Read the model definition and answer for the solid it produces. Units are mm, in the model's axes. Face numbers are marked on the shaded views. A direction names the side the tool comes from. Give positions to 0.01 mm unless a question says otherwise; leave off trailing zeros. Order: outer loops, then holes, each group sorted by start corner. A loop starts at its lowest first (then second) coordinate and runs counter-clockwise, first axis right, second up.
Item 1: A cutting plane is placed at A-A (x = -49). Write down the section's boundary in (y, z), plus the area to 3 significant figures.
Item 2: A cutting plane is placed at D-D (x = -16.5). Write down the section's boundary in (y, z), plus the area to 3 significant figures.
Item 3: Given pin 1 Ø17.5 at (x, z) = (-11.5, -19.92) entering from -Y; pin 2 Ø10 at (y, z) = (3.5, -34.5) entering from -X; pin 3 Ø9 at (x, z) = (34.972, -25.9) entering from -Y, each flat-ended and moving along its own axis, determine where each tip first touches the part or whether it passes through.
Item 4: Find the intervals of material crossed by line 1 along Z through (x, y) = (-34.5, 6.25); line 2 along X through (y, z) = (20, -22), in increasing order.
Item 5: Which of the six approach directions +Z, -Z, +X, -X, +Y, -Y give full straight-line access (tool end or side, diameter ignored) to the marked faces 1 and 2?
Item 6: A cutting plane is placed at C-C (y = 6.25). State how many separate pieces and enclosed holes the cut face has, plus the area to 3 significant figures.
Item 7: A cutting plane is placed at B-B (z = 6). Write down the section's boundary in (x, y).
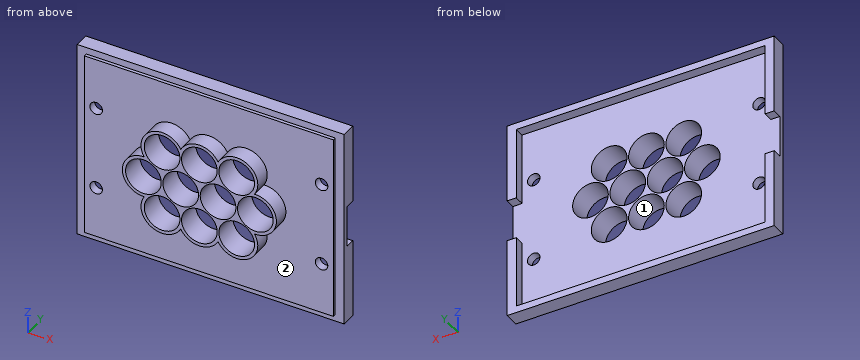
Autodesk Inventor part; units mm, degrees
ref_plane "YZ Plane" through (0, 0, 0) normal (1, 0, 0) x (0, 1, 0)
ref_plane "XZ Plane" through (0, 0, 0) normal (0, 1, 0) x (-1, 0, 0)
ref_plane "XY Plane" through (0, 0, 0) normal (0, 0, 1) x (1, 0, 0)
sketch "Sketch1" plane through (0, 0, 0) normal (0, 1, 0) x (-1, 0, 0)
  circle A0 centre (0, 0) radius 11
  line L0 (11, 0.0002) -> (12, 0.0002) construction
  circle A1 centre (23, 0) radius 11
  line L1 (34, 0) -> (35, 0) construction
  circle A2 centre (46, 0) radius 11
  line L2 (57, 0) -> (58, 0) construction
  circle A3 centre (69, 0) radius 11
  line L3 (34.5, 0) -> (34.5, -17.154) construction
  line L4 (34.5, 0) -> (34.5, 17.658) construction
  line L5 (55, 12.6387) -> (55, -13.5831) construction
  line L6 (55, 12.6387) -> (55, 17.658) construction
  line L7 (55, -13.5831) -> (55, -17.154) construction
  line L8 (11.5, 0.0002) -> (11.5, -16.2579) construction
  line L9 (11.5, 0.0002) -> (11.5, 19.9186) construction
  circle A4 centre (0, 0) radius 12 construction
  circle A5 centre (23, 0) radius 12 construction
  circle A6 centre (46, 0) radius 12 construction
  circle A7 centre (69, 0) radius 12 construction
  circle A8 centre (11.5, 19.9186) radius 11
  circle A9 centre (34.5, 19.9186) radius 11
  circle A10 centre (11.5, -19.9186) radius 11
  circle A11 centre (57.5, 19.9186) radius 11
  circle A12 centre (57.5, -19.9186) radius 12 construction
  circle A13 centre (34.5, -19.9186) radius 12 construction
  circle A14 centre (11.5, 19.9186) radius 12 construction
  circle A15 centre (34.5, 19.9186) radius 12 construction
  circle A16 centre (57.5, 19.9186) radius 12 construction
  line L10 (11.5, 19.9186) -> (57.5, 19.9186) construction
  arc A17 (2.3131, -12.7926) -> (0.5, -12.9904) centre (0, 0) ccw construction
  circle A18 centre (11.5, 19.9186) radius 13 construction
  circle A19 centre (34.5, 19.9186) radius 13 construction
  circle A20 centre (57.5, 19.9186) radius 13 construction
  circle A21 centre (69, 0) radius 13 construction
  circle A22 centre (57.5, -19.9186) radius 13 construction
  circle A23 centre (34.5, -19.9186) radius 13 construction
  arc A24 (0.5, 12.9904) -> (0.5, -12.9904) centre (0, 0) ccw
  line L11 (57.5, -19.9186) -> (11.5, -19.9186) construction
  circle A25 centre (11.5, -19.9186) radius 13 construction
  arc A26 (0.5, -12.9904) -> (23, -25.9808) centre (11.5, -19.9186) ccw
  arc A27 (23, -25.9808) -> (46, -25.9808) centre (34.5, -19.9186) ccw
  arc A28 (46, -25.9808) -> (68.5, -12.9904) centre (57.5, -19.9186) ccw
  arc A29 (68.5, -12.9904) -> (68.5, 12.9904) centre (69, 0) ccw
  arc A30 (68.5, 12.9904) -> (46, 25.9808) centre (57.5, 19.9186) ccw
  arc A31 (46, 25.9808) -> (23, 25.9808) centre (34.5, 19.9186) ccw
  arc A32 (23, 25.9808) -> (0.5, 12.9904) centre (11.5, 19.9186) ccw
  circle A33 centre (11.5, -19.9186) radius 12 construction
  circle A34 centre (34.5, -19.9186) radius 11
  circle A35 centre (57.5, -19.9186) radius 11
  dimension "d0" = 22
  dimension "d6" = 22
  dimension "d1" = 1
  dimension "d2" = 22
  dimension "d3" = 1
  dimension "d4" = 22
  dimension "d5" = 1
  dimension "d7" = 24
  dimension "d8" = 24
  dimension "d9" = 24
  dimension "d10" = 24
  dimension "d11" = 22
  dimension "d12" = 22
  dimension "d16" = 22
  dimension "d17" = 22
  dimension "d19" = 24
  dimension "d21" = 24
  dimension "d22" = 24
  dimension "d23" = 24
  dimension "d25" = 26
  dimension "d27" = 26
  dimension "d28" = 26
  dimension "d29" = 26
  dimension "d30" = 26
  dimension "d31" = 26
  dimension "d32" = 26
  dimension "d33" = 26
  dimension "d67" = 24
  dimension "d71" = 24
  dimension "d72" = 22
  dimension "d73" = 22
extrude "Extrusion1" add sketch "Sketch1" along normal blind 15
sketch "Sketch2" plane through (0, 15, 0) normal (0, 1, 0) x (1, 0, 0)
  circle A0 centre (-23, 0) radius 11
  circle A1 centre (-46, 0) radius 11
  line L0 (-35, 0) -> (-34, 0) construction
  line L1 (-111.2, 57.65) -> (42.2, 57.65)
  line L2 (42.2, 57.65) -> (42.2, -57.65)
  line L3 (42.2, -57.65) -> (-111.2, -57.65)
  line L4 (-111.2, -57.65) -> (-111.2, 57.65)
  line L5 (-111.2, 57.65) -> (42.2, -57.65) construction
  line L6 (42.2, 57.65) -> (-111.2, -57.65) construction
  arc A2 (-46, 25.9808) -> (-68.5, 12.9904) centre (-57.5, 19.9186) ccw
  arc A3 (-23, 25.9808) -> (-46, 25.9808) centre (-34.5, 19.9186) ccw
  arc A4 (-0.5, 12.9904) -> (-23, 25.9808) centre (-11.5, 19.9186) ccw
  arc A5 (-0.5, -12.9904) -> (-0.5, 12.9904) centre (0, 0) ccw
  arc A6 (-23, -25.9808) -> (-0.5, -12.9904) centre (-11.5, -19.9186) ccw
  arc A7 (-46, -25.9808) -> (-23, -25.9808) centre (-34.5, -19.9186) ccw
  arc A8 (-68.5, -12.9904) -> (-46, -25.9808) centre (-57.5, -19.9186) ccw
  arc A9 (-68.5, 12.9904) -> (-68.5, -12.9904) centre (-69, 0) ccw
  arc A10 (-69, 13) -> (-68.5, -12.9904) centre (-69, 0) ccw
  arc A11 (-46, 25.9808) -> (-68.5, 12.9904) centre (-57.5, 19.9186) ccw
  arc A12 (-23, 25.9808) -> (-46, 25.9808) centre (-34.5, 19.9186) ccw
  arc A13 (-0.5, 12.9904) -> (-23, 25.9808) centre (-11.5, 19.9186) ccw
  arc A14 (-0.5, -12.9904) -> (-0.5, 12.9904) centre (0, 0) ccw
  arc A15 (-23, -25.9808) -> (-0.5, -12.9904) centre (-11.5, -19.9186) ccw
  arc A16 (-46, -25.9808) -> (-23, -25.9808) centre (-34.5, -19.9186) ccw
  arc A17 (-68.5, -12.9904) -> (-46, -25.9808) centre (-57.5, -19.9186) ccw
  arc A18 (-68.5, 12.9904) -> (-68.5, -12.9904) centre (-69, 0) ccw
  point P0 (-34.5, 0)
  dimension "d36" = 115.3
  dimension "d37" = 153.4
extrude "Extrusion2" add sketch "Sketch2" against normal blind 5 contours L1 L2 L3 L4
sketch "Sketch3" plane through (0, 15, 0) normal (0, 1, 0) x (1, 0, 0)
  line L0 (42.2, 57.65) -> (-111.2, 57.65)
  line L1 (42.2, -57.65) -> (42.2, 57.65)
  line L2 (-111.2, -57.65) -> (42.2, -57.65)
  line L3 (-111.2, 57.65) -> (-111.2, -57.65)
  line L4 (-111.2, -57.65) -> (42.2, -57.65)
  line L5 (42.2, -57.65) -> (42.2, 57.65)
  line L6 (42.2, 57.65) -> (-111.2, 57.65)
  line L7 (-111.2, 57.65) -> (-111.2, -57.65)
  circle A0 centre (-57.5, -19.9186) radius 11
  circle A1 centre (-11.5, 19.9186) radius 11
  circle A2 centre (-34.5, -19.9186) radius 11
  circle A3 centre (-11.5, -19.9186) radius 11
  circle A4 centre (-69, 0) radius 11
  circle A5 centre (-46, 0) radius 11
  circle A6 centre (-23, 0) radius 11
  circle A7 centre (0, 0) radius 11
  line L8 (-116.8026, 61.8611) -> (47.8026, 61.8611)
  line L9 (47.8026, 61.8611) -> (47.8026, -61.8611)
  line L10 (47.8026, -61.8611) -> (-116.8026, -61.8611)
  line L11 (-116.8026, -61.8611) -> (-116.8026, 61.8611)
  line L12 (-116.8026, 61.8611) -> (47.8026, -61.8611) construction
  line L13 (47.8026, 61.8611) -> (-116.8026, -61.8611) construction
  line L14 (-111.2, -57.65) -> (42.2, -57.65)
  line L15 (42.2, -57.65) -> (42.2, 57.65)
  line L16 (42.2, 57.65) -> (-111.2, 57.65)
  line L17 (-111.2, 57.65) -> (-111.2, -57.65)
  line L18 (-111.2, -57.65) -> (42.2, 57.65) construction
  line L19 (42.2, -57.65) -> (-111.2, 57.65) construction
  point P0 (-34.5, 0)
extrude "Extrusion3" add sketch "Sketch3" along normal blind 6 and the other way blind 3 contours L8 L9 L10 L11
sketch "Sketch4" plane through (0, 15, 0) normal (0, 1, 0) x (1, 0, 0)
  line L0 (-111.2, -57.65) -> (42.2, -57.65)
  line L1 (42.2, -57.65) -> (42.2, 57.65)
  line L2 (42.2, 57.65) -> (-111.2, 57.65)
  line L3 (-111.2, 57.65) -> (-111.2, -57.65)
  circle A0 centre (-57.5, -19.9186) radius 11
  circle A1 centre (-11.5, 19.9186) radius 11
  circle A2 centre (-34.5, -19.9186) radius 11
  circle A3 centre (-11.5, -19.9186) radius 11
  circle A4 centre (-69, 0) radius 11
  circle A5 centre (-46, 0) radius 11
  circle A6 centre (-23, 0) radius 11
  circle A7 centre (0, 0) radius 11
  line L4 (-111.2, 57.65) -> (-103.972, 57.65) construction
  line L5 (-103.972, 57.65) -> (-103.972, 25.9) construction
  line L6 (-103.972, 25.9) -> (-111.2, 25.9) construction
  line L7 (-111.2, 25.9) -> (-111.2, 57.65) construction
  line L8 (42.2, 57.65) -> (34.972, 57.65) construction
  line L9 (34.972, 57.65) -> (34.972, 25.9) construction
  line L10 (34.972, 25.9) -> (42.2, 25.9) construction
  line L11 (42.2, 25.9) -> (42.2, 57.65) construction
  line L12 (-111.2, -57.65) -> (-103.972, -57.65) construction
  line L13 (-103.972, -57.65) -> (-103.972, -25.9) construction
  line L14 (-103.972, -25.9) -> (-111.2, -25.9) construction
  line L15 (-111.2, -25.9) -> (-111.2, -57.65) construction
  line L16 (42.2, -25.9) -> (34.972, -25.9) construction
  line L17 (34.972, -25.9) -> (34.972, -57.65) construction
  line L18 (34.972, -57.65) -> (42.2, -57.65) construction
  line L19 (42.2, -57.65) -> (42.2, -25.9) construction
  circle A8 centre (-103.972, 25.9) radius 3.865
  circle A9 centre (34.972, 25.9) radius 3.865
  circle A10 centre (34.972, -25.9) radius 3.865
  circle A11 centre (-103.972, -25.9) radius 3.865
  dimension "d56" = 7.73
  dimension "d57" = 7.73
  dimension "d58" = 7.73
  dimension "d59" = 7.73
  dimension "d62" = 7.228
  dimension "d63" = 31.75
  dimension "d64" = 7.228
  dimension "d65" = 7.228
  dimension "d66" = 31.75
extrude "Extrusion4" cut sketch "Sketch4" against normal through all contours A8 | A9 | A10 | A11
sketch "Sketch5" plane through (-116.8026, 12, 61.8611) normal (-1, 0, 0) x (0, 0, 1)
  line L0 (-74.8611, -12) -> (-74.8611, -2)
  line L1 (-48.8611, -12) -> (-48.8611, -2)
  line L2 (-119.5111, 3) -> (-4.2111, 3)
  line L3 (-123.7222, 9) -> (0, 9)
  line L4 (-74.8611, 3) -> (-48.8611, 3)
  line L5 (-48.8611, 3) -> (-48.8611, 9)
  line L6 (-48.8611, 9) -> (-74.8611, 9)
  line L7 (-74.8611, 9) -> (-74.8611, 3)
  point P0 (-61.8611, -12)
extrude "Extrusion5" cut sketch "Sketch5" against normal through all
properties part number "CELLCASE21700_3DPrint"
Response values:
1. outline: (0, -29.75) - (10, -29.75) - (10, -57.65) - (12, -57.65) - (12, -61.86) - (21, -61.86) - (21, -57.65) - (15, -57.65) - (15, -26.9) - (0, -26.9) - close; (0, -12.94) - (15, -12.94) - (15, -10.58) - (0, -10.58) - close; (0, 10.58) - (15, 10.58) - (15, 12.94) - (0, 12.94) - close; (0, 26.9) - (15, 26.9) - (15, 57.65) - (21, 57.65) - (21, 61.86) - (12, 61.86) - (12, 57.65) - (10, 57.65) - (10, 29.75) - (0, 29.75) - close
1. area: 511 mm2
2. outline: (0, -31.92) - (10, -31.92) - (10, -57.65) - (12, -57.65) - (12, -61.86) - (21, -61.86) - (21, -57.65) - (15, -57.65) - (15, -29.72) - (0, -29.72) - close; (0, -10.12) - (15, -10.12) - (15, -8.87) - (0, -8.87) - close; (0, 8.87) - (15, 8.87) - (15, 10.12) - (0, 10.12) - close; (0, 29.72) - (15, 29.72) - (15, 57.65) - (21, 57.65) - (21, 61.86) - (12, 61.86) - (12, 57.65) - (10, 57.65) - (10, 31.92) - (0, 31.92) - close
2. area: 437 mm2
3. pin 1: passes through
3. pin 2: stops at x = -66.29
3. pin 3: stops at y = 10
4. line 1: z = -32.92 to -30.92, -8.92 to 8.92, 30.92 to 32.92
4. line 2: x = -116.8 to -111.2, 42.2 to 47.8
5. face 1: +Y, -Y
5. face 2: -Y
6. separate pieces: 1
6. enclosed holes: 10
6. area: 1,050 mm2
7. outline: (-116.8, 12) - (-111.2, 12) - (-111.2, 10) - (-80.53, 10) - (-80.53, 0) - (-78.22, 0) - (-78.22, 15) - (-116.8, 15) - close; (-59.78, 0) - (-55.22, 0) - (-55.22, 15) - (-59.78, 15) - close; (-36.78, 0) - (-32.22, 0) - (-32.22, 15) - (-36.78, 15) - close; (-13.78, 0) - (-9.22, 0) - (-9.22, 15) - (-13.78, 15) - close; (9.22, 0) - (11.53, 0) - (11.53, 10) - (42.2, 10) - (42.2, 12) - (47.8, 12) - (47.8, 15) - (9.22, 15) - close
